Drawing for the job (mm, zero at the part's lowest x, y, z). A direction names the side the tool comes from. Round coordinates to 2 decimals unless told otherwise and drop trailing zeros. Loops run counter-clockwise (first coordinate to the right, second up) from the corner with the lowest first, then second, coordinate; pieces in that order, holes last.
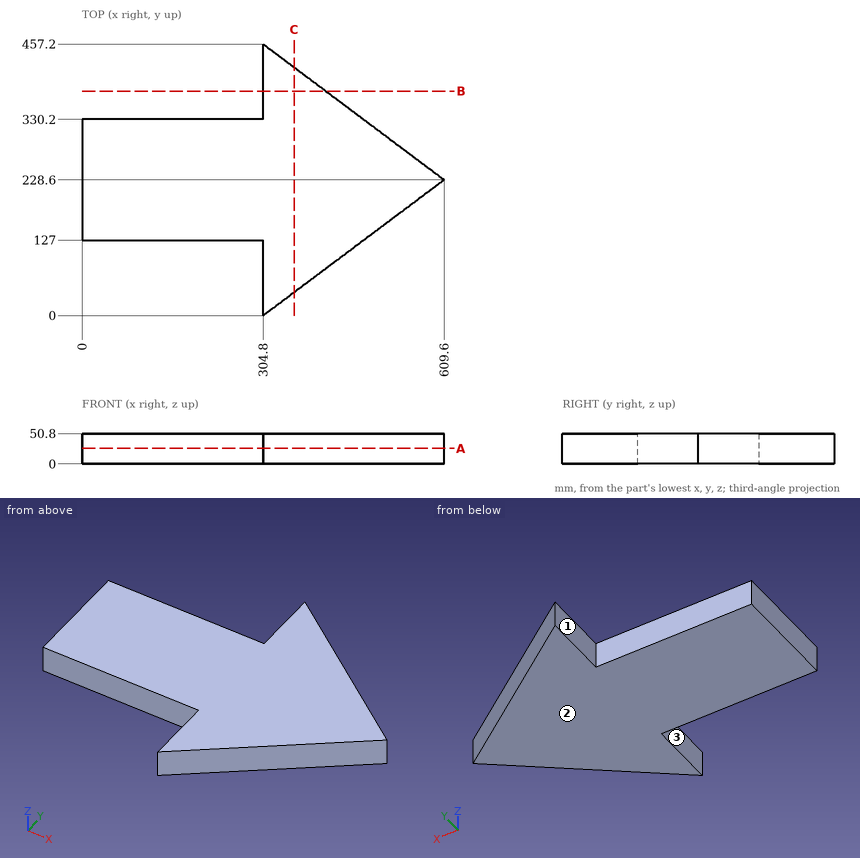
Q1. Slice it at B-B on y = 378. Give the cut face in (x, z), plus the area to 3 significant figures.
Q2. Tool access for the marked faces 1, 2 and 3: list every direction of +Z, -Z, +X, -X, +Y, -Y with a clear straight run to the whole face (end or side of a thin tool).
Q3. Probe line 1 (Y direction, x = 195.5, z = 25.5); line 2 (Y direction, x = 377.5, z = 25.5) (3 decimals); line 3 (X direction, y = 115, z = 9.5). List the from-to ranges inside material, lowest first.
Q4. Flat gauge pins, fed straight in: P1, Ø1, axis at x = 180.5, z = 9.5, coming from the -Y side; P2, Ø6, axis at x = 263, z = 15.5, coming from the +Y side; P3, Ø4, axis at x = 486, z = 7.5, coming from the -Y side. Where does each tip first touch, or does it go through?
Q5. Slice it at C-C on x = 357. Give the cut face in (y, z), plus the area to 3 significant figures.
Q6. Slice it at A-A on z = 26. Give the cut face in (x, y), plus the area to 3 significant figures.
Reply:
1. outline: (304.8, 0) - (410.4, 0) - (410.4, 50.8) - (304.8, 50.8) - close
1. area: 5,360 mm2
2. face 1: +Z, -Z, -X, +Y
2. face 2: -Z, +X, -X, +Y, -Y
2. face 3: +Z, -Z, -X, -Y
3. line 1: y = 127 to 330.2
3. line 2: y = 54.525 to 402.675
3. line 3: x = 304.8 to 458.13
4. P1: stops at y = 127
4. P2: stops at y = 330.2
4. P3: stops at y = 134.4
5. outline: (39.15, 0) - (418.05, 0) - (418.05, 50.8) - (39.15, 50.8) - close
5. area: 19,200 mm2
6. outline: (0, 127) - (304.8, 127) - (304.8, 0) - (609.6, 228.6) - (304.8, 457.2) - (304.8, 330.2) - (0, 330.2) - close
6. area: 132,000 mm2
